```python
from build123d import *

# Parameters (mm, degrees)
SKETCH3_W           = 4
SKETCH3_H           = 12.8
CUT_EXTRUDE1_DEPTH  = 60.170622077
SKETCH4_W           = 19.5
SKETCH4_H           = 2
SKETCH4_W_2         = 1.5
SKETCH4_H_2         = 14.3
BOSS_EXTRUDE1_DEPTH = 1
BOSS_EXTRUDE2_DEPTH = 0.6
SKETCH6_W           = 19.5
SKETCH6_H           = 3.3
BOSS_EXTRUDE3_DEPTH = 1
FILLET1_R           = 3


with BuildPart() as part:
    # Sketch1 → Loft1 section 0
    with BuildSketch(Plane(origin=(0, 0, 0), x_dir=(1, 0, 0), z_dir=(0, 1, 0))):
        with BuildLine():
            Line((-48.15, -34.3), (48.15, -34.3))
            Line((48.15, -34.3), (48.15, 34.3))
            Line((48.15, 34.3), (-48.15, 34.3))
            Line((-48.15, 34.3), (-48.15, -34.3))
        make_face()
    # Sketch2 → Loft1 section 1
    with BuildSketch(Plane(origin=(0, 2.5, 0), x_dir=(1, 0, 0), z_dir=(0, 1, 0))):
        with BuildLine():
            Line((-46.65, -32.8), (46.65, -32.8))
            Line((46.65, -32.8), (46.65, 32.8))
            Line((46.65, 32.8), (-46.65, 32.8))
            Line((-46.65, 32.8), (-46.65, -32.8))
        make_face()
    loft()

    # Sketch3 → Cut-Extrude1 (cut, through all)
    with BuildSketch(Plane.XZ):
        with Locations((46.15, 0)):
            Rectangle(SKETCH3_W, SKETCH3_H)
    extrude(amount=-CUT_EXTRUDE1_DEPTH, mode=Mode.SUBTRACT)

    # Sketch4 → Boss-Extrude1 (add)
    with BuildSketch(Plane.XZ):
        with Locations((21, 32)):
            Rectangle(SKETCH4_W, SKETCH4_H)
        with Locations((21, -32)):
            Rectangle(SKETCH4_W, SKETCH4_H)
        with Locations((-46.1, 0)):
            Rectangle(SKETCH4_W_2, SKETCH4_H_2)
    extrude(amount=BOSS_EXTRUDE1_DEPTH)

    # Sketch5 → Boss-Extrude2 (add)
    with BuildSketch(Plane.XZ.offset(1)):
        Polygon((-50.55, -11.25), (-45.35, -11.25), (-45.35, 11.25), (-50.55, 11.25), (-50.55, 1), (-48.55, 1), (-48.55, -1), (-50.55, -1), align=None)
    extrude(amount=BOSS_EXTRUDE2_DEPTH)

    # Sketch6 → Boss-Extrude3 (add)
    with BuildSketch(Plane.XZ.offset(1)):
        with Locations((21, 32.65)):
            Rectangle(SKETCH6_W, SKETCH6_H)
        with Locations((21, -32.65)):
            Rectangle(SKETCH6_W, SKETCH6_H)
    extrude(amount=BOSS_EXTRUDE3_DEPTH)

    # Fillet1
    # the kernel refuses this fillet: 3 mm, written as the material it takes off along each edge
    with BuildSketch(Plane(origin=(-50.76627907, -4.360465116, 36.91627907), x_dir=(-0.23537960143467007, -0.3922993357244589, -0.8892118276421003), z_dir=(0.4574957109978059, 0.7624928516630279, -0.45749571099781455)), Plane(origin=(50.76627907, -4.360465116, -36.91627907), x_dir=(0.2353796014346717, -0.39229933572445586, 0.8892118276421013), z_dir=(-0.4574957109978127, 0.7624928516630248, 0.4574957109978127)), Plane(origin=(-50.76627907, -4.360465116, -36.91627907), x_dir=(0.8892118276421047, -0.39229933572444886, -0.23537960143466988), z_dir=(0.4574957109978059, 0.7624928516630279, 0.45749571099781455))) as fillet1_piece_1:
        with BuildLine():
            CenterArc((FILLET1_R * 0.762492851663, -FILLET1_R), FILLET1_R, 90, 74.650522983)
            Line((-FILLET1_R * 0.201836343087, -FILLET1_R * 0.735294117647), (0, 0))
            Line((0, 0), (FILLET1_R * 0.762492851663, 0))
        make_face()
    extrude(amount=14.716112037, mode=Mode.SUBTRACT)
    with BuildSketch(Plane(origin=(50.76627907, -4.360465116, 36.91627907), x_dir=(0.2353796014346717, -0.39229933572445586, -0.8892118276421013), z_dir=(-0.4574957109978127, 0.7624928516630248, -0.4574957109978127))) as fillet1_piece_2:
        with BuildLine():
            CenterArc((FILLET1_R * 0.762492851663, FILLET1_R), FILLET1_R, 195.349477017, 74.650522983)
            Line((-FILLET1_R * 0.201836343087, FILLET1_R * 0.735294117647), (0, 0))
            Line((0, 0), (FILLET1_R * 0.762492851663, 0))
        make_face()
    extrude(amount=14.716112037, mode=Mode.SUBTRACT)


solid = part.part
```
Here's how the part is built. I have some questions about the finished solid (model axes, mm). A direction names the side the tool comes from. Round coordinates to 2 decimals unless told otherwise and drop trailing zeros. Answer as CSV lines item,"result".
Item 1: For pin 1 (0.7 mm diameter, centred on y = -1, z = 0, fed in from -X); pin 2 (0.5 mm diameter, centred on x = 23, y = -0.5, fed in from -Z); pin 3 (0.6 mm diameter, centred on y = -1, z = -33.5, fed in from +X); pin 4 (1 mm diameter, centred on x = -10.5, y = -1, fed in from -Z), each with a flat end and sliding along its axis, tell me the tip position at first contact or that it passes through.
From the geometry:
pin 1,"x = -48.55"
pin 2,"z = -33"
pin 3,"x = 30.75"
pin 4,"through"
Item 2: Please list where these lines run through material, in increasing order: L1, parallel to Z at x = 17, y = -0.7; L2, parallel to Y at x = -39.5, z = 31; L3, parallel to X at y = -1.2, z = -5. Write a range as [from, to].
From the geometry:
L1,"[-33, -31], [31, 33]"
L2,"[0, 2.5]"
L3,"[-50.55, -45.35]"
Item 3: Which directions (+Z, -Z, +X, -X, +Y, -Y) give clear straight access to the entire face, cutting with the end or side of a thin tool? Please do faces 5 (the flat face through (30.75, -1, -32)), 6 (the flat face through (46, 1, 6.4)), 7 (the flat face through (21, -1, 31)), 8 (the flat face through (11.25, -1, -32)).
From the geometry:
face 5,"+Z, -Z, +X, -Y"
face 6,"+X, +Y, -Y"
face 7,"+X, -X, -Y"
face 8,"+Z, -Z, -X, -Y"
Item 4: We'd pull the mould along Z, two halves only. Please class faces 1 (the cylindrical face through (-46.58, 1.39, -32.77)), 2 (the cylindrical face through (46.58, 1.39, 32.77)), 3 (the flat face through (21, -2, 33)), 4 (the flat face through (44.15, 1, 0)): +Z half, -Z half, draft (parallel to the pull), parting line (faces both ways), or undercut.
From the geometry:
face 1,"-Z half"
face 2,"+Z half"
face 3,"draft"
face 4,"undercut"
